The listing builds one solid part. Answer for the finished solid, in the listing's coordinates (mm). Give positions to 0.01 mm unless a question says otherwise; leave off trailing zeros. Order: outer loops, then holes, each group sorted by start corner. A loop starts at its lowest first (then second) coordinate and runs counter-clockwise, first axis right, second up. Notation, with made-up numbers: (9, -3.75) - (56, -3.75) arc R8 ccw to (56, 2.25) - close; hole circle Ø4 at (74, -18.75). An arc over 180 degrees is marked (long way). Answer in a Markdown table with one row per item. Add a question column.
Autodesk Inventor part; units mm, degrees
ref_plane "Work Plane1" through (6, 0, 0) normal (0, 0.5, 0.866) x (1, 0, 0)
ref_plane "YZ Plane" through (0, 0, 0) normal (1, 0, 0) x (0, 1, 0)
ref_plane "XZ Plane" through (0, 0, 0) normal (0, 1, 0) x (-1, 0, 0)
sketch "Sketch1" plane through (0, 0, 0) normal (0, 0, 1) x (1, 0, 0)
  line L0 (0, 0) -> (8.8333, 0)
  line L1 (12, 1.1547) -> (12, 2)
  line L2 (12, 2) -> (0, 2)
  line L3 (12, 1.1547) -> (9.5, 1.1547)
  line L4 (9.5, 1.1547) -> (8.8333, 0)
  line L5 (0, -0.4) -> (0, 2.4)
  line L6 (0, 2) -> (0, 0)
  dimension "d0" = 2.5
  dimension "d1" = 60
  dimension "d2" = 4
  dimension "d3" = 2.3094
  dimension "d5" = 12
revolve "Body" add sketch "Sketch1" angle 360 about axis through (0, 0, 0) along (1, 0, 0)
chamfer "Chamfer1" distance 0.4294 angle 60 1 edges at (12, -2, 0) measured on face at (12, 1.6877, -0.2517)
sketch "Sketch2" plane through (12, 0, 0) normal (1, 0, 0) x (0, 0, -1)
  circle A0 centre (0, 0) radius 1.1547
  line L0 (-0.5774, 1) -> (0.5774, 1)
  line L1 (0.5774, 1) -> (1.1547, 0)
  line L2 (1.1547, 0) -> (0.5774, -1)
  line L3 (0.5774, -1) -> (-0.5774, -1)
  line L4 (-0.5774, -1) -> (-1.1547, 0)
  line L5 (-1.1547, 0) -> (-0.5774, 1)
  point P0 (0, 0)
  point P1 (0, 0)
extrude "Slot" add sketch "Sketch2" against normal up to next contours L1 A0 | A0 L2 | L0 A0 | A0 L3 | L5 A0 | A0 L4
thread "Thread"
chamfer "Chamfer2" distance 0.4294 angle 60 1 edges at (0, -2, 0) measured on face at (3.7521, 1.9935, -0.1609)
ref_plane "Work Plane1" through (6, 0, 0) normal (0, 0.5, 0.866) x (1, 0, 0)
equation "\"d0\" = INTI"
equation "\"d2\" = NND"
equation "\"d3\" = 1.1547 * SW"
equation "\"d5\" = NLG"
equation "\"d7\" = -0.5 * GD1 + 0.5 * NND"
equation "\"d8\" = FAWI"
equation "\"d29\" = -0.5 * GD1 + 0.5 * NND"
equation "\"d11\" = NLG"
equation "\"d13\" = -0.5 * GD1 + 0.5 * NND"
equation "\"d14\" = FAWI"
equation "\"d30\" = -0.5 * GD1 + 0.5 * NND"
equation "\"NND\" = 4"
equation "\"NLG\" = 12"
equation "\"INTI\" = 2.5"
equation "\"FAWI\" = 60deg"
equation "\"SW\" = 2"
equation "\"GD1\" = THREADDIA - 1.2269 * PTC"
equation "\"FAWI1\" = 45deg"
equation "\"GUL\" = 0.61345 * PTC"
equation "\"SPD\" = 2"
equation "\"TOA\" = 30deg"
equation "\"THREADDIA\" = 4"
equation "\"PTC\" = 0.7"
equation "\"GAL\" = 0.61345 * PTC"
equation "\"E0\" = 1.155 * SW"
properties part number "AS 1421 - M4 x 12 Flat Point" material "Steel, Mild"
(1) Straight lines are drawn through the part: line 1 (X direction, y = 0, z = 1.5); line 2 (Y direction, x = 4, z = -0.5); line 3 (Y direction, x = 3.75, z = -0.4). For each, find the intervals that lie inside material, in ascending order.
(2) The mould has two halves that part along Y. Classify faces 1 (the face through (0, 0, 0)), 2 (the face through (10.72, 0.49, 0.87)), 3 (the face through (6, 0, 2)): +Y half, -Y half, draft (parallel to the pull), parting line (faces both ways), or undercut.
(3) Find section B-B, the plane x = 9.25. Write down the section's boundary in (y, z).
(4) Find section A-A, the plane x = 5. Write down the section's boundary in (y, z), plus the area to 3 significant figures.
(5) This flat-tipped pin is pushed along its axis until it touches: P1, Ø1.5, axis at x = 2.5, y = 1.5, coming from the +Z side. Where does it stop, or does it pass through?
Answer key:
| question | item | result |
|---|---|---|
| 1 | line 1 | 0.14 to 12 |
| 1 | line 2 | -1.94 to 1.94 |
| 1 | line 3 | -1.96 to 1.96 |
| 2 | face 1 | draft |
| 2 | face 2 | undercut |
| 2 | face 3 | parting line |
| 3 | outline | circle Ø4 at (0, 0); hole circle Ø1.44 at (0, 0) |
| 4 | outline | circle Ø4 at (0, 0) |
| 4 | area | 12.6 mm² |
| 5 | P1 | z = 1.85 |
